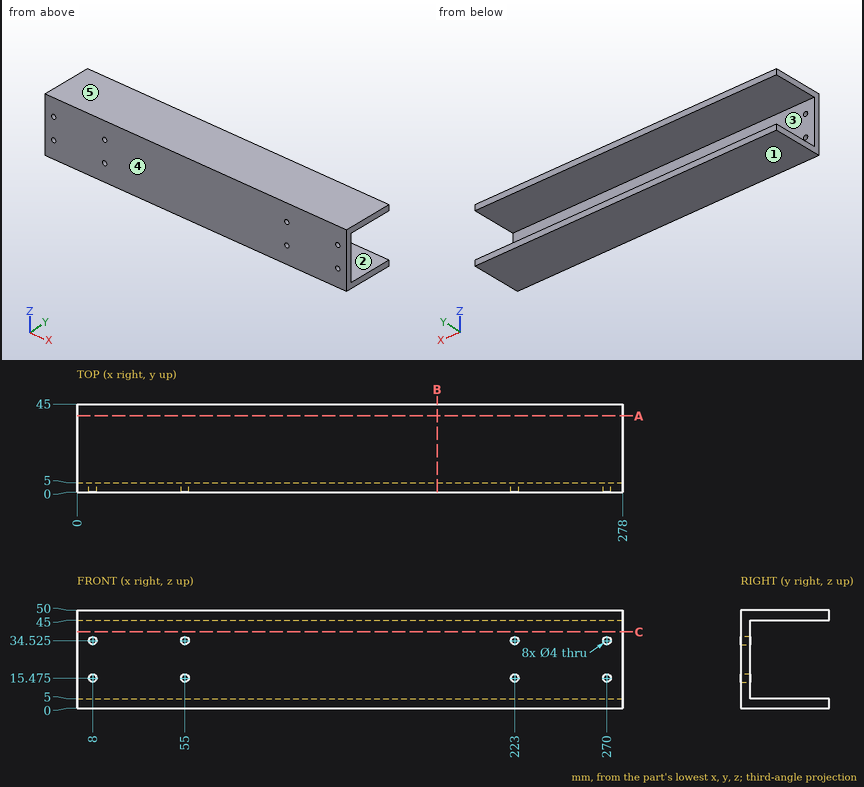
Can you work these out from the drawing? Everything is in mm from the part's minimum corner. A direction names the side the tool comes from. Give positions to 0.01 mm unless a question says otherwise; leave off trailing zeros. Loops run counter-clockwise (first coordinate to the right, second up) from the corner with the lowest first, then second, coordinate; pieces in that order, holes last. Notation, with made-up numbers: (-32, -25.75) -> (3, -25.75) arc R20 cw to (3, -0.75) -> close; hole circle Ø11 at (34.5, 89). An arc over 180 degrees is marked (long way). Return JSON: item names as keys, results as strings.
Q1. We'd pull the mould along Z, two halves only. Please class the marked faces 3, 4 and 5: released by +Z, released by -Z, zero draft, split by the parting line, or undercut.
Checks:
{"face 3": "undercut", "face 4": "zero draft", "face 5": "released by +Z"}
Q2. I want a section at B-B, the plane x = 183.5. List the corners of the cut face in (y, z) for me.
Checks:
{"outline": "(0, 0) -> (45, 0) -> (45, 5) -> (5, 5) -> (5, 45) -> (45, 45) -> (45, 50) -> (0, 50) -> close"}
Q3. I need wall thicknesses on probe 1 along Z at (x, y) = (270, 2) (3 decimals); probe 2 along Z at (x, y) = (71.5, 17.5); probe 3 along Y at (x, z) = (171, 16.5). Which ranges of each line are inside material? Lowest first, please.
Checks:
{"probe 1": "z = 0 to 13.475, 17.475 to 32.525, 36.525 to 50", "probe 2": "z = 0 to 5, 45 to 50", "probe 3": "y = 0 to 5"}
Q4. For pin 1 Ø20 at (x, z) = (89.5, 17) entering from +Y; pin 2 Ø6.5 at (x, z) = (8, 15.475) entering from -Y, each with a flat end and sliding along its axis, tell me the tip position at first contact or that it passes through.
Checks:
{"pin 1": "stops at y = 5", "pin 2": "stops at y = 0"}
Q5. I want a section at A-A, the plane y = 39. List the corners of the cut face in (x, z) for me.
Checks:
{"outline": "(0, 0) -> (278, 0) -> (278, 5) -> (0, 5) -> close; (0, 45) -> (278, 45) -> (278, 50) -> (0, 50) -> close"}
Q6. I want a section at C-C, the plane z = 39. List the corners of the cut face in (x, y) for me, then the cut area to 3 significant figures.
Checks:
{"outline": "(0, 0) -> (278, 0) -> (278, 5) -> (0, 5) -> close", "area": "1,390 mm2"}
Q7. On a 3-axis mill with a long thin cutter (end or side, diameter ignored), from which of +Z, -Z, +X, -X, +Y, -Y can I reach the whole of each face in a straight line? I mean the marked faces 1 and 2. Say none if no direction works.
Checks:
{"face 1": "-Z, +X, -X, +Y, -Y", "face 2": "+X, -X, +Y"}
